CAD build for the part. Positions are in the model's coordinates, mm. Coordinates: 2 decimals unless noted, no trailing zeros. Order: outer loops, then holes, each group sorted by start corner. A loop starts at its lowest first (then second) coordinate and runs counter-clockwise, first axis right, second up. Notation, with made-up numbers: (6.25, 77) - (56.25, 77) arc R14 cw to (56.25, 93) - close; hole circle Ø9 at (-39, -3). An arc over 180 degrees is marked (long way). Write each question's results on one line, items separated by ' | '. Start each with the question number.
Q1. Band-saw the part on B-B, the plane x = 237.5. Write the cut outline in (y, z), then the cut area to 3 significant figures.
Q2. Band-saw the part on C-C, the plane y = 17.75. Write the cut outline in (x, z), then the cut area to 3 significant figures.
Q3. Band-saw the part on A-A, the plane z = -12.25. Write the cut outline in (x, y).
Q4. Wall check: probe 1 along Y at (x, z) = (237.5, -11); probe 2 along X at (y, z) = (11, -8.5); probe 3 along X at (y, z) = (6.25, -22.25). Give the ranges that are in metal, low to high.
Q5. Pull direction Y, two halves, no side cores. Call faces 1 (the flat face through (123, 25, -13)), 2 (the cylindrical face through (244.89, 9.44, -12.32)), 3 (the flat face through (123, 12, -25)): released by +Y, released by -Y, zero draft, split by the parting line, or undercut.
```python
from build123d import *

# Parameters (mm, degrees)
SKETCH1_W           = 250
SKETCH1_H           = 25
BOSS_EXTRUDE1_DEPTH = 25
SKETCH2_R           = 8
CUT_EXTRUDE1_DEPTH  = 26


with BuildPart() as part:
    # Sketch1 → Boss-Extrude1 (new body)
    with BuildSketch(Plane(origin=(0, 0, 0), x_dir=(1, 0, 0), z_dir=(0, 1, 0))):
        with Locations((125, 12.5)):
            Rectangle(SKETCH1_W, SKETCH1_H)
    extrude(amount=BOSS_EXTRUDE1_DEPTH)

    # Sketch2 → Cut-Extrude1 (cut, through all)
    with BuildSketch(Plane.XY):
        with Locations((237.5, 12.5)):
            Circle(SKETCH2_R)
    extrude(amount=-CUT_EXTRUDE1_DEPTH, mode=Mode.SUBTRACT)


solid = part.part
```
Results below:
1) outline: (0, -25) - (4.5, -25) - (4.5, 0) - (0, 0) - close; (20.5, -25) - (25, -25) - (25, 0) - (20.5, 0) - close | area: 225 mm²
2) outline: (0, -25) - (231.46, -25) - (231.46, 0) - (0, 0) - close; (243.54, -25) - (250, -25) - (250, 0) - (243.54, 0) - close | area: 5,950 mm²
3) outline: (0, 0) - (250, 0) - (250, 25) - (0, 25) - close; hole circle Ø16 at (237.5, 12.5)
4) probe 1: y = 0 to 4.5, 20.5 to 25 | probe 2: x = 0 to 229.64, 245.36 to 250 | probe 3: x = 0 to 232.51, 242.49 to 250
5) face 1: released by +Y | face 2: undercut | face 3: zero draft
